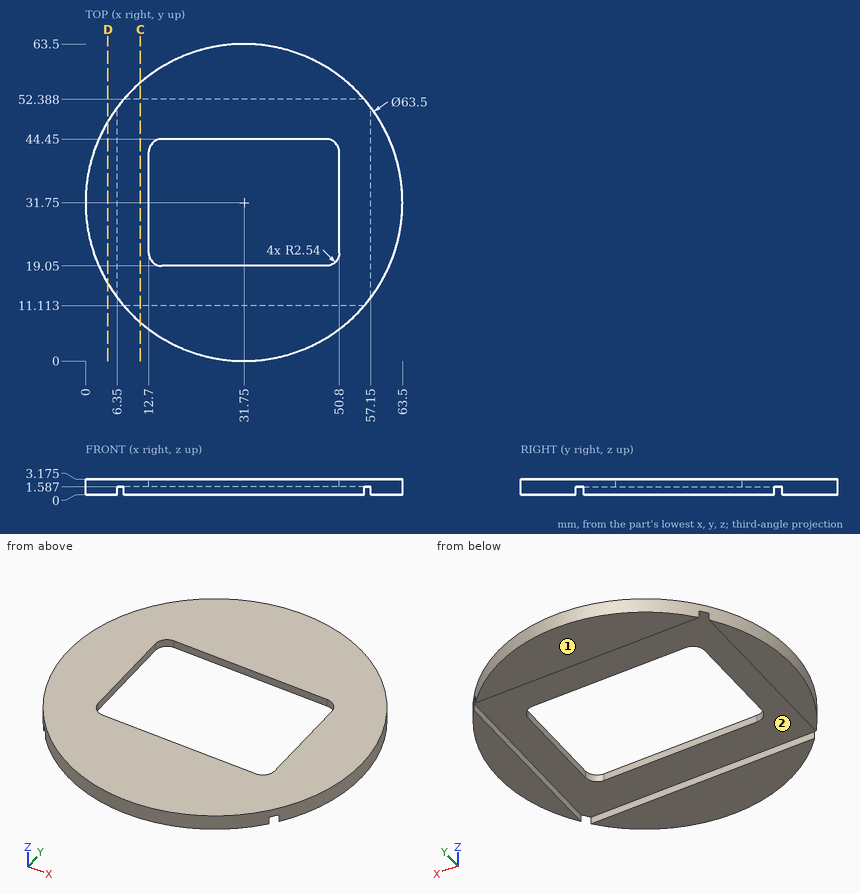
Verification items for this drawing (mm, ordinates from the low corner). Round coordinates to 2 decimals unless told otherwise and drop trailing zeros. Loops run counter-clockwise (first coordinate to the right, second up) from the corner with the lowest first, then second, coordinate; pieces in that order, holes last. Notation, with made-up numbers: (40.5, -36) -> (67.5, -36) arc R21 cw to (67.5, -9) -> close; hole circle Ø1 at (-25, 29.25). An arc over 180 degrees is marked (long way). Write item = value, one per line. Start each with the question number.
1) Sectioned sample at D-D, the plane x = 4.5. Record the cut outline in (y, z) (1 decimal).
2) Release check for a two-part mould opening along X. For the marked faces 1 and 2 record: released by +X, released by -X, zero draft, split by the parting line, or undercut.
3) Thickness scan on probe 1 along Y at (x, z) = (32, 1.45); probe 2 along X at (y, z) = (32, 0.2); probe 3 along X at (y, z) = (20, 2.15) (1 decimal). Record the ranges inside material, lowest first.
4) Sectioned sample at C-C, the plane x = 11. Record the cut outline in (y, z) (1 decimal).
5) Gauge pin test, flat ends, axial feed: pin 1 Ø1.3 at (x, z) = (21, 0.5) entering from +Y; pin 2 Ø0.8 at (y, z) = (36.5, 0.5) entering from -X; pin 3 Ø0.8 at (x, z) = (26.5, 0.5) entering from -Y; pin 4 Ø8 at (x, y) = (48, 24) entering from +Z (1 decimal). Record the tip position at first contact, or that the pin passes through.
Results are:
q1.outline = (15.5, 0) -> (48, 0) -> (48, 3.2) -> (15.5, 3.2) -> close
q2.face_1 = zero draft
q2.face_2 = undercut
q3.probe_1 = 0 to 11.11, 52.39 to 63.5
q3.probe_2 = 0 to 6.35, 57.15 to 63.5
q3.probe_3 = 2.3 to 13.3, 50.2 to 61.2
q4.outline = (7.7, 0) -> (11.1, 0) -> (11.1, 1.6) -> (52.4, 1.6) -> (52.4, 0) -> (55.8, 0) -> (55.8, 3.2) -> (7.7, 3.2) -> close
q5.pin_1 = 61.85
q5.pin_2 = 0.3
q5.pin_3 = 0.37
q5.pin_4 = 3.2
